from build123d import *

# Parameters (mm, degrees)
F1_DEPTH      = 1.5
F2_W          = 19
F2_H          = 15
F3_DEPTH      = 4.5
F4_W          = 9
F4_H          = 3
F5_DEPTH      = 12.5
F6_W          = 9
F6_H          = 2
F7_DEPTH      = 1.2
F8_W          = 9
F8_H          = 2
F9_DEPTH      = 1.3
F10_R         = 2
F11_T1_DEPTH  = 8
F11_T3_DEPTH  = 2.5
F11_T5_DEPTH  = 8
F11_T7_DEPTH  = 15
F11_T9_DEPTH  = 12.8412291828
F11_T11_DEPTH = 12.8412291828
F11_T14_ANGLE = 90
F11_T16_ANGLE = 90
F11_T18_ANGLE = 90
F11_T20_ANGLE = 90
F11_T22_ANGLE = 90
F11_T24_ANGLE = 90
F11_T26_ANGLE = 90
F11_T28_ANGLE = 90
F12_T1_DEPTH  = 9
F14_DEPTH     = 12.5


# Not quite as in the source:
# - a fillet or chamfer that OpenCascade refuses, or shapes differently, is made with other operations: its cross-section is extruded or revolved along the edge and cut away or added


with BuildPart() as f1:
    # F0 (on Top) → F1 (new body)
    with BuildSketch(Plane.XY):
        with BuildLine():
            Line((12.5, 9.5), (-12.5, 9.5))
            ThreePointArc((-12.5, 9.5), (-13.9142135624, 8.9142135624), (-14.5, 7.5))
            Line((-14.5, 7.5), (-14.5, -7.5))
            ThreePointArc((-14.5, -7.5), (-13.9142135624, -8.9142135624), (-12.5, -9.5))
            Line((-12.5, -9.5), (12.5, -9.5))
            ThreePointArc((12.5, -9.5), (13.9142135624, -8.9142135624), (14.5, -7.5))
            Line((14.5, -7.5), (14.5, 7.5))
            ThreePointArc((14.5, 7.5), (13.9142135624, 8.9142135624), (12.5, 9.5))
        make_face()
    extrude(amount=F1_DEPTH)

    # F2 (on face) → F3 (join)
    with BuildSketch(Plane.XY.offset(1.5)):
        Rectangle(F2_W, F2_H)
    extrude(amount=F3_DEPTH)

    # F4 (on Front) → F5 (cut, symmetric)
    with BuildSketch(Plane.XZ):
        with Locations((0, 2.5)):
            Rectangle(F4_W, F4_H)
    extrude(amount=F5_DEPTH, both=True, mode=Mode.SUBTRACT)

    # F6 (on face) → F7 (cut)
    with BuildSketch(Plane.XZ.offset(7.5)):
        with Locations((0, 5)):
            Rectangle(F6_W, F6_H)
    extrude(amount=-F7_DEPTH, mode=Mode.SUBTRACT)

    # F8 (on face) → F9 (cut)
    with BuildSketch(Plane(origin=(0, 7.5, 0), x_dir=(-1, 0, 0), z_dir=(0, 1, 0))):
        with Locations((0, 5)):
            Rectangle(F8_W, F8_H)
    extrude(amount=-F9_DEPTH, mode=Mode.SUBTRACT)

    # F10
    f10_edges = [f1.edges().sort_by_distance(p)[0] for p in [
        (9.5, 0, 6),
        (-9.5, 0, 6),
    ]]
    fillet(f10_edges, radius=F10_R)

    # F11: fillet of radius 2 on 18 edges, made by hand

    # F11_s2 → F11_t1 (cut)
    with BuildSketch(Plane.YZ.offset(-0.5)):
        with BuildLine():
            ThreePointArc((7.5, 4), (6.9142135624, 5.4142135624), (5.5, 6))
            Line((5.5, 6), (7.5, 6))
            Line((7.5, 6), (7.5, 4))
        make_face()
        with BuildLine():
            ThreePointArc((-5.5, 6), (-6.9142135624, 5.4142135624), (-7.5, 4))
            Line((-7.5, 4), (-7.5, 6))
            Line((-7.5, 6), (-5.5, 6))
        make_face()
    extrude(amount=F11_T1_DEPTH, mode=Mode.SUBTRACT)

    # F11_s4 → F11_t3 (cut)
    with BuildSketch(Plane.XY.offset(1.5)):
        with BuildLine():
            ThreePointArc((7.5, 7.5), (8.9142135624, 6.9142135624), (9.5, 5.5))
            Line((9.5, 5.5), (9.5, 7.5))
            Line((9.5, 7.5), (7.5, 7.5))
        make_face()
        with BuildLine():
            ThreePointArc((-7.5, 7.5), (-8.9142135624, 6.9142135624), (-9.5, 5.5))
            Line((-9.5, 5.5), (-9.5, 7.5))
            Line((-9.5, 7.5), (-7.5, 7.5))
        make_face()
        with BuildLine():
            ThreePointArc((9.5, -5.5), (8.9142135624, -6.9142135624), (7.5, -7.5))
            Line((7.5, -7.5), (9.5, -7.5))
            Line((9.5, -7.5), (9.5, -5.5))
        make_face()
        with BuildLine():
            ThreePointArc((-7.5, -7.5), (-8.9142135624, -6.9142135624), (-9.5, -5.5))
            Line((-9.5, -5.5), (-9.5, -7.5))
            Line((-9.5, -7.5), (-7.5, -7.5))
        make_face()
    extrude(amount=F11_T3_DEPTH, mode=Mode.SUBTRACT)

    # F11_s6 → F11_t5 (cut)
    with BuildSketch(Plane.YZ.offset(-7.5)):
        with BuildLine():
            ThreePointArc((5.5, 6), (6.9142135624, 5.4142135624), (7.5, 4))
            Line((7.5, 4), (7.5, 6))
            Line((7.5, 6), (5.5, 6))
        make_face()
        with BuildLine():
            ThreePointArc((-5.5, 6), (-6.9142135624, 5.4142135624), (-7.5, 4))
            Line((-7.5, 4), (-7.5, 6))
            Line((-7.5, 6), (-5.5, 6))
        make_face()
    extrude(amount=F11_T5_DEPTH, mode=Mode.SUBTRACT)

    # F11_s8 → F11_t7 (cut)
    with BuildSketch(Plane.XZ.offset(-7.5)):
        with BuildLine():
            ThreePointArc((12.5635083269, 1.5), (13.7882531983, 1.0811388301), (14.5, 0))
            Line((14.5, 0), (14.5, 1.5))
            Line((14.5, 1.5), (12.5635083269, 1.5))
        make_face()
        with BuildLine():
            ThreePointArc((-12.5635083269, 1.5), (-13.7882531983, 1.0811388301), (-14.5, 0))
            Line((-14.5, 0), (-14.5, 1.5))
            Line((-14.5, 1.5), (-12.5635083269, 1.5))
        make_face()
    extrude(amount=F11_T7_DEPTH, mode=Mode.SUBTRACT)

    # F11_s10 → F11_t9 (cut)
    with BuildSketch(Plane.YZ.offset(-0.3412291828)):
        with BuildLine():
            ThreePointArc((-7.5635083269, 1.5), (-8.7882531983, 1.0811388301), (-9.5, 0))
            Line((-9.5, 0), (-9.5, 1.5))
            Line((-9.5, 1.5), (-7.5635083269, 1.5))
        make_face()
        with BuildLine():
            ThreePointArc((7.5635083269, 1.5), (8.7882531983, 1.0811388301), (9.5, 0))
            Line((9.5, 0), (9.5, 1.5))
            Line((9.5, 1.5), (7.5635083269, 1.5))
        make_face()
    extrude(amount=F11_T9_DEPTH, mode=Mode.SUBTRACT)

    # F11_s12 → F11_t11 (cut)
    with BuildSketch(Plane.YZ.offset(-12.5)):
        with BuildLine():
            ThreePointArc((-9.5, 0), (-8.7882531983, 1.0811388301), (-7.5635083269, 1.5))
            Line((-7.5635083269, 1.5), (-9.5, 1.5))
            Line((-9.5, 1.5), (-9.5, 0))
        make_face()
        with BuildLine():
            ThreePointArc((9.5, 0), (8.7882531983, 1.0811388301), (7.5635083269, 1.5))
            Line((7.5635083269, 1.5), (9.5, 1.5))
            Line((9.5, 1.5), (9.5, 0))
        make_face()
    extrude(amount=F11_T11_DEPTH, mode=Mode.SUBTRACT)

    # F11_s13 → F11_t14 (revolve, cut)
    with BuildSketch(Plane.YZ.offset(7.5)):
        with BuildLine():
            ThreePointArc((7.5, 4), (6.9142135624, 5.4142135624), (5.5, 6))
            Line((5.5, 6), (7.5, 6))
            Line((7.5, 6), (7.5, 4))
        make_face()
    revolve(axis=Axis((7.5, 7.5, 4), (0, 1, 0)), revolution_arc=F11_T14_ANGLE, mode=Mode.SUBTRACT)

    # F11_s15 → F11_t16 (revolve, cut)
    with BuildSketch(Plane.YZ.offset(-7.5)):
        with BuildLine():
            ThreePointArc((5.5, 6), (6.9142135624, 5.4142135624), (7.5, 4))
            Line((7.5, 4), (7.5, 6))
            Line((7.5, 6), (5.5, 6))
        make_face()
    revolve(axis=Axis((-7.5, 7.5, 4), (0, -1, 0)), revolution_arc=F11_T16_ANGLE, mode=Mode.SUBTRACT)

    # F11_s17 → F11_t18 (revolve, cut)
    with BuildSketch(Plane.YZ.offset(7.5)):
        with BuildLine():
            ThreePointArc((-5.5, 6), (-6.9142135624, 5.4142135624), (-7.5, 4))
            Line((-7.5, 4), (-7.5, 6))
            Line((-7.5, 6), (-5.5, 6))
        make_face()
    revolve(axis=Axis((7.5, -7.5, 4), (0, 1, 0)), revolution_arc=F11_T18_ANGLE, mode=Mode.SUBTRACT)

    # F11_s19 → F11_t20 (revolve, cut)
    with BuildSketch(Plane.YZ.offset(-7.5)):
        with BuildLine():
            ThreePointArc((-7.5, 4), (-6.9142135624, 5.4142135624), (-5.5, 6))
            Line((-5.5, 6), (-7.5, 6))
            Line((-7.5, 6), (-7.5, 4))
        make_face()
    revolve(axis=Axis((-7.5, -7.5, 4), (0, -1, 0)), revolution_arc=F11_T20_ANGLE, mode=Mode.SUBTRACT)

    # F11_s21 → F11_t22 (revolve, cut)
    with BuildSketch(Plane.YZ.offset(-12.5)):
        with BuildLine():
            ThreePointArc((7.5635083269, 1.5), (8.7882531983, 1.0811388301), (9.5, 0))
            Line((9.5, 0), (9.5, 1.5))
            Line((9.5, 1.5), (7.5635083269, 1.5))
        make_face()
    revolve(axis=Axis((-12.5, 7.5, 1.5), (0, 0, 1)), revolution_arc=F11_T22_ANGLE, mode=Mode.SUBTRACT)

    # F11_s23 → F11_t24 (revolve, cut)
    with BuildSketch(Plane.XZ.offset(-7.5)):
        with BuildLine():
            ThreePointArc((12.5635083269, 1.5), (13.7882531983, 1.0811388301), (14.5, 0))
            Line((14.5, 0), (14.5, 1.5))
            Line((14.5, 1.5), (12.5635083269, 1.5))
        make_face()
    revolve(axis=Axis((12.5, 7.5, 1.5), (0, 0, 1)), revolution_arc=F11_T24_ANGLE, mode=Mode.SUBTRACT)

    # F11_s25 → F11_t26 (revolve, cut)
    with BuildSketch(Plane.XZ.offset(7.5)):
        with BuildLine():
            ThreePointArc((-12.5635083269, 1.5), (-13.7882531983, 1.0811388301), (-14.5, 0))
            Line((-14.5, 0), (-14.5, 1.5))
            Line((-14.5, 1.5), (-12.5635083269, 1.5))
        make_face()
    revolve(axis=Axis((-12.5, -7.5, 1.5), (0, 0, 1)), revolution_arc=F11_T26_ANGLE, mode=Mode.SUBTRACT)

    # F11_s27 → F11_t28 (revolve, cut)
    with BuildSketch(Plane.YZ.offset(12.5)):
        with BuildLine():
            ThreePointArc((-7.5635083269, 1.5), (-8.7882531983, 1.0811388301), (-9.5, 0))
            Line((-9.5, 0), (-9.5, 1.5))
            Line((-9.5, 1.5), (-7.5635083269, 1.5))
        make_face()
    revolve(axis=Axis((12.5, -7.5, 1.5), (0, 0, 1)), revolution_arc=F11_T28_ANGLE, mode=Mode.SUBTRACT)

    # F12: fillet of radius 1 on 4 edges, made by hand

    # F12_s2 → F12_t1 (cut)
    with BuildSketch(Plane.YZ.offset(-4.5)):
        with BuildLine():
            ThreePointArc((-6.3, 5), (-6.0071067812, 4.2928932188), (-5.3, 4))
            Line((-5.3, 4), (-6.3, 4))
            Line((-6.3, 4), (-6.3, 5))
        make_face()
        with BuildLine():
            ThreePointArc((5.2, 4), (5.9071067812, 4.2928932188), (6.2, 5))
            Line((6.2, 5), (6.2, 4))
            Line((6.2, 4), (5.2, 4))
        make_face()
        with BuildLine():
            ThreePointArc((6.2, 5), (5.9071067812, 5.7071067812), (5.2, 6))
            Line((5.2, 6), (5.2, 6.1))
            ThreePointArc((5.2, 6.1), (5.5, 6.1), (6.235, 5.9671743695))
            Line((6.235, 5.9671743695), (6.3, 5.8734993995))
            Line((6.3, 5.8734993995), (6.3, 5))
            Line((6.3, 5), (6.2, 5))
        make_face()
        with BuildLine():
            ThreePointArc((-5.3, 6), (-6.0071067812, 5.7071067812), (-6.3, 5))
            Line((-6.3, 5), (-6.4, 5))
            Line((-6.4, 5), (-6.4, 5.833030278))
            Line((-6.4, 5.833030278), (-6.34, 5.9246817919))
            ThreePointArc((-6.34, 5.9246817919), (-5.5, 6.1), (-5.3, 6.1))
            Line((-5.3, 6.1), (-5.3, 6))
        make_face()
    extrude(amount=F12_T1_DEPTH, mode=Mode.SUBTRACT)

    # F13 (on Right) → F14 (cut, symmetric)
    with BuildSketch(Plane.YZ):
        Polygon((-10, 6.9632698071), (0, 5.2), (10, 6.9632698071), align=None)
    extrude(amount=F14_DEPTH, both=True, mode=Mode.SUBTRACT)


solid = f1.part
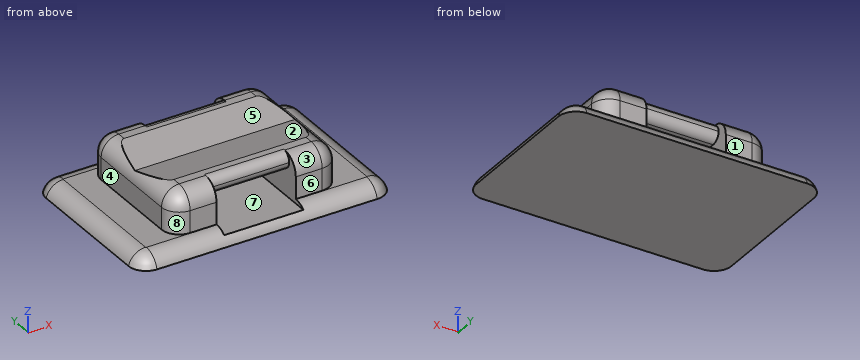
Input: part model. Units: mm. Frame: model coordinates. Face numbers are marked on the shaded views. A direction names the side the tool comes from. Round coordinates to 2 decimals unless told otherwise and drop trailing zeros. Order: outer loops, then holes, each group sorted by start corner. A loop starts at its lowest first (then second) coordinate and runs counter-clockwise, first axis right, second up.
1. Material intervals for line 1 (X direction, y = -4.25, z = 3.4); line 2 (X direction, y = 4.25, z = 4.1); line 3 (Z direction, x = 4.25, y = 7.25), sorted ascending.
The answers:
line 1: x = -9.5 to -4.5, 4.5 to 9.5
line 2: x = -9.5 to 9.5
line 3: z = 0 to 1
2. Pin query (flat end, axial travel): P1, Ø0.8, axis at y = -1.5, z = 3, coming from the +X side; P2, Ø3, axis at x = 5.5, z = 2.5, coming from the +Y side; P3, Ø0.8, axis at x = 6.5, z = 2.5, coming from the -Y side. Return the tip coordinate at first contact, or that it passes through.
The answers:
P1: stops at x = 9.5
P2: stops at y = 8.89
P3: stops at y = -7.5
3. Cut plane C-C, the plane z = 2.35. Output: boundary loops of the cut face in (x, y).
The answers:
outline: (-9.5, -5.5) arc R2 ccw to (-7.5, -7.5) - (-4.5, -7.5) - (-4.5, 7.5) - (-7.5, 7.5) arc R2 ccw to (-9.5, 5.5) - close; (4.5, -7.5) - (7.5, -7.5) arc R2 ccw to (9.5, -5.5) - (9.5, 5.5) arc R2 ccw to (7.5, 7.5) - (4.5, 7.5) - close
4. Mould query, pull axis Y, two halves, no side actions, for the marked faces 1, 2, 3 and 4. Classes: released by +Y, released by -Y, zero draft, split by the parting line, or undercut.
The answers:
face 1: released by +Y
face 2: undercut
face 3: released by -Y
face 4: zero draft
5. Set-up query: the marked faces 5, 6, 7 and 8. Return all of +Z, -Z, +X, -X, +Y, -Y with unobstructed straight access to the full face (end or side cutting, diameter ignored); none if empty.
The answers:
face 5: +Z, +X, -X
face 6: +Z, +X, -X, -Y
face 7: +Y, -Y
face 8: +Z, -X, -Y
6. Cut plane D-D, the plane x = 6.75. Output: boundary loops of the cut face in (y, z).
The answers:
outline: (-9.5, 0) - (9.5, 0) arc R2 ccw to (7.56, 1.5) - (7.5, 1.5) - (7.5, 4) arc R2 ccw to (5.5, 6) - (4.54, 6) - (0, 5.2) - (-4.54, 6) - (-5.5, 6) arc R2 ccw to (-7.5, 4) - (-7.5, 1.5) - (-7.56, 1.5) arc R2 ccw to start
7. Cut plane B-B, the plane y = -5. Output: boundary loops of the cut face in (x, z), then the cut area to 3 significant figures.
The answers:
outline: (-14.5, 0) - (14.5, 0) arc R2 ccw to (12.56, 1.5) - (9.5, 1.5) - (9.5, 4) arc R2 ccw to (7.5, 6) - (-7.5, 6) arc R2 ccw to (-9.5, 4) - (-9.5, 1.5) - (-12.56, 1.5) arc R2 ccw to start; hole (-4.5, 1) - (4.5, 1) - (4.5, 4) - (-4.5, 4) - close
area: 98.8 mm2
8. Cut plane A-A, the plane x = 1.75. Output: boundary loops of the cut face in (y, z), then the cut area to 3 significant figures.
The answers:
outline: (-9.5, 0) - (9.5, 0) arc R2 ccw to (8.89, 1) - (-8.89, 1) arc R2 ccw to start; (-5.3, 4) - (5.2, 4) arc R1 ccw to (5.2, 6) - (4.54, 6) - (0, 5.2) - (-4.54, 6) - (-5.3, 6) arc R1 ccw to start
area: 39.0 mm2
